Geometry: final body of the model. Coordinates: model frame, mm. Give positions to 0.01 mm unless a question says otherwise; leave off trailing zeros. Order: outer loops, then holes, each group sorted by start corner. A loop starts at its lowest first (then second) coordinate and runs counter-clockwise, first axis right, second up. Notation, with made-up numbers: (-27.5, 40) -> (-11.5, 40) arc R32 cw to (-11.5, 67) -> close; hole circle Ø9 at (61, 5). An arc over 180 degrees is marked (long way). One line per question, with ' | ' between items. Start each with the question number.
(1) Section A-A (y = 41). Return loops of the section in (x, z), then the cut area to 3 significant figures.
(2) Ray query, L1, parallel to Z at x = 4.5, y = 6; L2, parallel to Y at x = 2.5, z = -63. Return the intervals inside material, ascending.
(3) Section B-B (z = 0). Return loops of the section in (x, y).
(4) First-contact query: pin 1 Ø4.5 at (y, z) = (-66.675, -66.675) entering from +X; pin 2 Ø2.5 at (y, z) = (-66.675, 0) entering from +X. Flat tips, straight axial feed; report the tip coordinate or a pass-through.
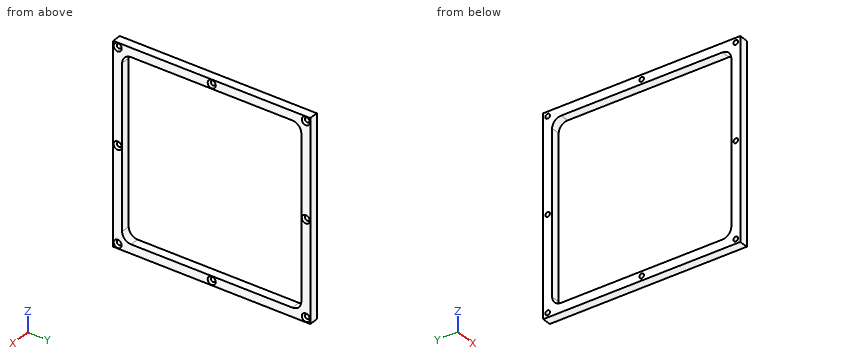
Autodesk Inventor part; units mm, degrees
ref_plane "YZ Plane" through (0, 0, 0) normal (1, 0, 0) x (0, 1, 0)
ref_plane "XZ Plane" through (0, 0, 0) normal (0, 1, 0) x (-1, 0, 0)
ref_plane "XY Plane" through (0, 0, 0) normal (0, 0, 1) x (1, 0, 0)
sketch "Sketch1" plane through (0, 0, 0) normal (1, 0, 0) x (0, 1, 0)
  line L0 (-69.85, -69.85) -> (69.85, -69.85)
  line L1 (69.85, -69.85) -> (69.85, 69.85)
  line L2 (69.85, 69.85) -> (-69.85, 69.85)
  line L3 (-69.85, 69.85) -> (-69.85, -69.85)
  line L4 (-69.85, -69.85) -> (69.85, 69.85) construction
  line L5 (69.85, -69.85) -> (-69.85, 69.85) construction
  point P0 (0, 0)
  dimension "d0" = 139.7
  dimension "d1" = 139.7
extrude "Extrusion1" add sketch "Sketch1" along normal blind 6.35
sketch "Sketch6" plane through (6.35, 0, 0) normal (1, 0, 0) x (0, 0, -1)
  line L0 (69.85, -69.85) -> (69.85, 69.85)
  line L1 (69.85, 69.85) -> (-69.85, 69.85)
  line L2 (-69.85, 69.85) -> (-69.85, -69.85)
  line L3 (-69.85, -69.85) -> (69.85, -69.85)
  point P0 (0, 0)
  point P1 (-66.675, -66.675)
  point P2 (-66.675, 0)
  dimension "d45" = 3.175
  dimension "d46" = 3.175
  dimension "d61" = 69.85
hole "Hole4" at (6.35, -66.675, 66.675) at (6.35, 0, 66.675) direction (-1, 0, 0) diameter 3.2766 end through all countersink diameter 5.715 countersink angle 82
pattern_circular "Circular Pattern1" count 4 over 360 about axis through (-10, 0, 0) along (1, 0, 0) of "Hole4"
sketch "Sketch7" plane through (6.35, 0, 0) normal (1, 0, 0) x (0, 0, -1)
  circle A0 centre (-66.675, 66.675) radius 2.8575
  circle A1 centre (66.675, 66.675) radius 2.8575
  circle A2 centre (66.675, -66.675) radius 2.8575
  circle A3 centre (-66.675, -66.675) radius 2.8575
  line L0 (69.85, -69.85) -> (69.85, 69.85)
  line L1 (69.85, 69.85) -> (-69.85, 69.85)
  line L2 (-69.85, 69.85) -> (-69.85, -69.85)
  line L3 (-69.85, -69.85) -> (69.85, -69.85)
  line L4 (-63.5, -63.5) -> (-63.5, 63.5)
  line L5 (-63.5, 63.5) -> (63.5, 63.5)
  line L6 (63.5, 63.5) -> (63.5, -63.5)
  line L7 (63.5, -63.5) -> (-63.5, -63.5)
  point P0 (0, 0)
  dimension "d57" = 6.35
extrude "Extrusion3" cut sketch "Sketch7" against normal through all contours L4 L5 L6 L7
fillet "Fillet1" radius 6.35 4 edges at (3.175, -63.5, -63.5) (3.175, 63.5, 63.5) (3.175, -63.5, 63.5) (3.175, 63.5, -63.5)
equation "\"d0\" = width + 2 * plasticThickness"
equation "\"d1\" = height + 2 * plasticThickness"
equation "\"d2\" = caseThickness"
equation "\"d57\" = caseThickness"
equation "\"d60\" = caseThickness"
equation "\"height\" = 127"
equation "\"width\" = 127"
equation "\"plasticThickness\" = 6.35"
equation "\"caseThickness\" = 6.35"
equation "\"alignmentGrooveDepth\" = 1.5875"
equation "\"alignmentGrooveClearance\" = 0.1016"
equation "\"aerogelHolderDepth\" = 49.022"
equation "\"depth\" = 203.2"
equation "\"mirrorAngle\" = 2.5deg"
equation "\"mirrorThickness\" = 3.175"
equation "\"fresnelThickness\" = 0.254"
equation "\"focalLength\" = 152.4"
equation "\"ior\" = 1.49"
equation "\"centerThickness\" = 1.27"
equation "\"fresnelAngle\" = 90deg"
equation "\"fresnelEffectiveDiameter\" = 152.4"
equation "\"frontPanelThickness\" = 1.5875"
equation "\"fresnelGrooveWidth\" = 1.778"
properties part number "frontClamp" material "Aluminum 6061"
Response:
1) outline: (0, -69.85) -> (6.35, -69.85) -> (6.35, -63.5) -> (0, -63.5) -> close; (0, 63.5) -> (6.35, 63.5) -> (6.35, 69.85) -> (0, 69.85) -> close | area: 80.6 mm^2
2) L1: z = -69.85 to -63.5, 63.5 to 69.85 | L2: y = -69.85 to -59.62, 59.62 to 69.85
3) outline: (0, -69.85) -> (6.35, -69.85) -> (6.35, -69.53) -> (4.95, -68.31) -> (0, -68.31) -> close; (0, -65.04) -> (4.95, -65.04) -> (6.35, -63.82) -> (6.35, -63.5) -> (0, -63.5) -> close; (0, 63.5) -> (6.35, 63.5) -> (6.35, 63.82) -> (4.95, 65.04) -> (0, 65.04) -> close; (0, 68.31) -> (4.95, 68.31) -> (6.35, 69.53) -> (6.35, 69.85) -> (0, 69.85) -> close
4) pin 1: stops at x = 5.65 | pin 2: passes through
